Input: dimensioned drawing with shaded views. Units: mm. Origin: part minimum x, y, z. Coordinates: 2 decimals unless noted, no trailing zeros. Loops run counter-clockwise (first coordinate to the right, second up) from the corner with the lowest first, then second, coordinate; pieces in that order, holes last. Notation, with made-up numbers: (74.5, 32.5) - (104.5, 32.5) arc R24 ccw to (104.5, 57.5) - close; hole circle Ø8 at (80.25, 84.5). An arc over 180 degrees is marked (long way). Put each result on its own line as item: value. Start each with the question number.
1) Contact query for flat-ended pins moving along their axis: pin 1 Ø0.9 at (y, z) = (1.5, 16) entering from +X; pin 2 Ø2.5 at (x, z) = (4, 3.5) entering from -Y; pin 3 Ø1.5 at (y, z) = (2, 35.5) entering from +X. Output: stop coordinate, or through.
2) Section A-A on z = 35. Output: boundary loops of the cut face in (x, y).
3) Section C-C on x = 4. Output: boundary loops of the cut face in (y, z), and give its area (3 significant figures).
4) Section B-B on x = 74.5. Output: boundary loops of the cut face in (y, z), and give its area (3 significant figures).
5) Section D-D on y = 1.95. Count the separate pieces of the cut face and the enclosed holes in it, and give its area (3 significant figures).
6) Material intervals for line 1 along Z through (x, y) = (91, 1.4); line 2 along Z through (x, y) = (82, 2.5); line 3 along X through (y, z) = (2.2, 3.5), sorted ascending. Write a range as from..to.
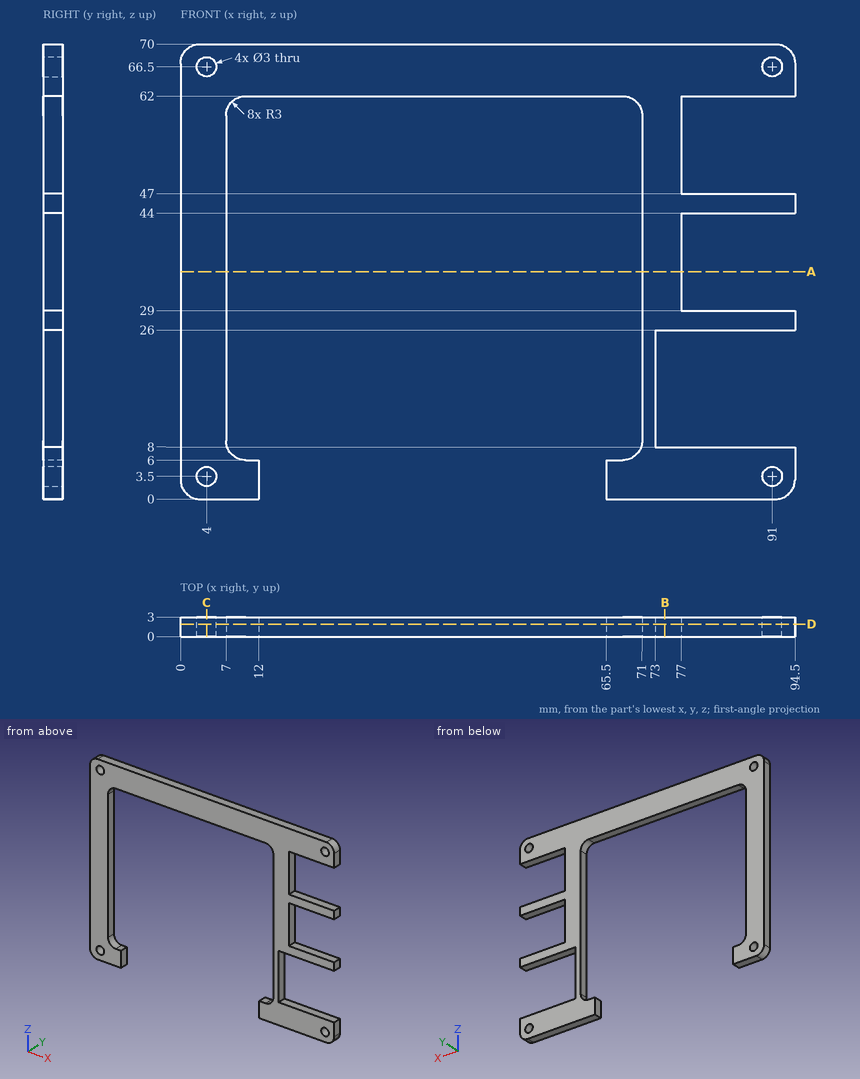
Answer block:
1. pin 1: stops at x = 73
1. pin 2: passes through
1. pin 3: stops at x = 77
2. outline: (0, 0) - (7, 0) - (7, 3) - (0, 3) - close; (71, 0) - (77, 0) - (77, 3) - (71, 3) - close
3. outline: (0, 0) - (3, 0) - (3, 2) - (0, 2) - close; (0, 5) - (3, 5) - (3, 65) - (0, 65) - close; (0, 68) - (3, 68) - (3, 70) - (0, 70) - close
3. area: 192 mm²
4. outline: (0, 0) - (3, 0) - (3, 8) - (0, 8) - close; (0, 26) - (3, 26) - (3, 70) - (0, 70) - close
4. area: 156 mm²
5. separate pieces: 1
5. enclosed holes: 4
5. area: 1,770 mm²
6. line 1: z = 0..2, 5..8, 26..29, 44..47, 62..65, 68..70
6. line 2: z = 0..8, 26..29, 44..47, 62..70
6. line 3: x = 0..2.5, 5.5..12, 65.5..89.5, 92.5..94.5
